Could you check a few things on this drawing? It's one solid part, dimensions in mm from its lowest x, y, z. Coordinates: 2 decimals unless noted, no trailing zeros. Order: outer loops, then holes, each group sorted by start corner. A loop starts at its lowest first (then second) coordinate and runs counter-clockwise, first axis right, second up. Notation, with made-up numbers: (-34, -15.75) - (-20, -15.75) arc R19 cw to (-20, -3.75) - close; hole circle Ø8 at (-36, 32). An arc over 180 degrees is marked (long way). Answer in a Markdown table with one row per item. Add a question column.
Item 1: I want a section at C-C (x = 50). Please give me the cut outline in (y, z), plus the area to 3 significant figures.
Item 2: I want a section at D-D (x = 8). Please give me the cut outline in (y, z), plus the area to 3 significant figures.
Item 3: Thinking about a two-plate mould opening in X: for the marked faces 1, 2, 3 and 4, which applies, +X half, -X half, draft (parallel to the pull), parting line (faces both ways), or undercut?
Item 4: I want a section at A-A (z = 56). Please give me the cut outline in (x, y).
Item 5: Will these pins go through, and if not, where does the flat tip stop? pin 1 Ø2.5 at (x, y) = (96.5, 5) entering from -Z; pin 2 Ø4 at (x, y) = (46, 6) entering from -Z; pin 3 Ø2 at (x, y) = (51, 1.5) entering from +Z.
Item 6: I want a section at B-B (y = 6.5). Please give me the cut outline in (x, z).
Item 7: If I drill on line 1 along X through (y, z) = (3.25, 21); line 2 along X through (y, z) = (3.5, 72); line 3 along X through (y, z) = (1.75, 24), over which ranges is the centre line in solid material (lowest first)? Write a range as from..to.
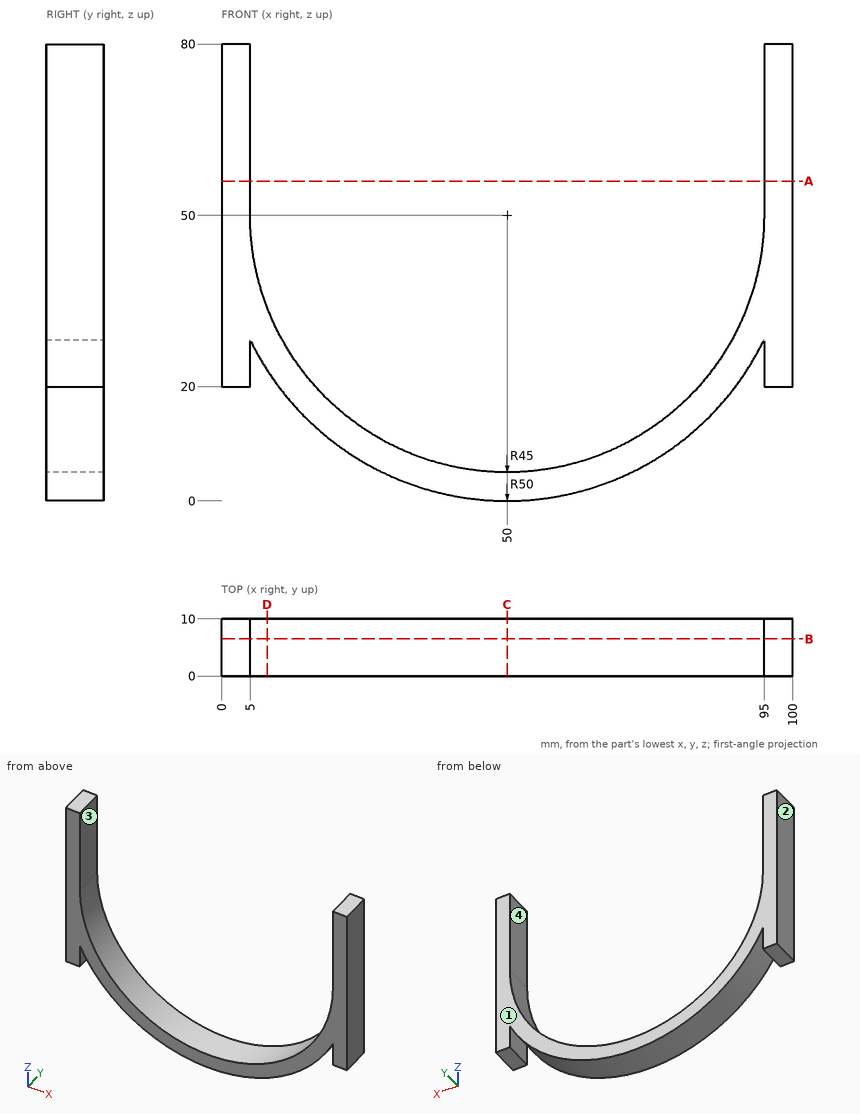
Values follow:
| question | item | result |
|---|---|---|
| 1 | outline | (0, 0) - (10, 0) - (10, 5) - (0, 5) - close |
| 1 | area | 50.0 mm^2 |
| 2 | outline | (0, 22.87) - (10, 22.87) - (10, 33.84) - (0, 33.84) - close |
| 2 | area | 110 mm^2 |
| 3 | face 1 | draft |
| 3 | face 2 | -X half |
| 3 | face 3 | undercut |
| 3 | face 4 | undercut |
| 4 | outline | (0, 0) - (5, 0) - (5, 10) - (0, 10) - close; (95, 0) - (100, 0) - (100, 10) - (95, 10) - close |
| 5 | pin 1 | stops at z = 20 |
| 5 | pin 2 | stops at z = 0.04 |
| 5 | pin 3 | stops at z = 5.04 |
| 6 | outline | (0, 20) - (5, 20) - (5, 28.21) arc R50 ccw to (95, 28.21) - (95, 20) - (100, 20) - (100, 80) - (95, 80) - (95, 50) arc R45 cw to (5, 50) - (5, 80) - (0, 80) - close |
| 7 | line 1 | x = 0..5, 9.27..15.59, 84.41..90.73, 95..100 |
| 7 | line 2 | x = 0..5, 95..100 |
| 7 | line 3 | x = 0..5, 7.29..13.27, 86.73..92.71, 95..100 |
